Drawing for the job (mm, zero at the part's lowest x, y, z). Give positions to 0.01 mm unless a question says otherwise; leave off trailing zeros.
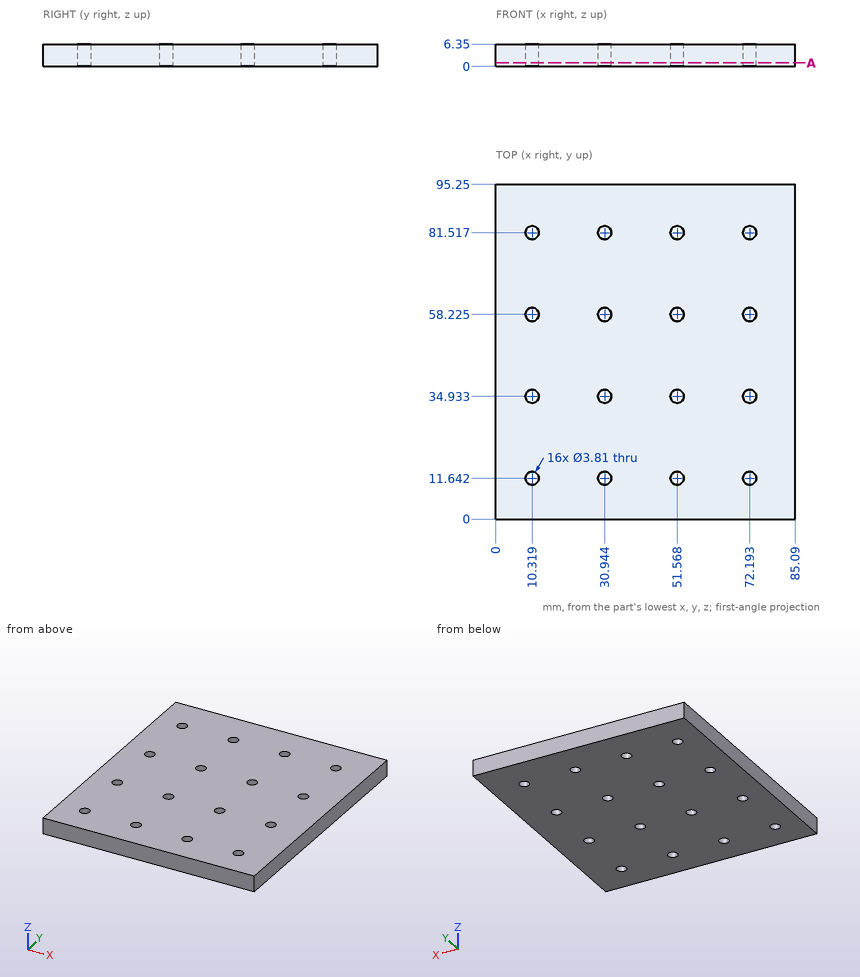
1. Slice it at A-A, the plane z = 1. State how many separate pieces and enclosed holes the cut face has, and give its area (3 significant figures).
Calculated:
separate pieces: 1
enclosed holes: 16
area: 7,920 mm2
2. Probe probe 1 along X at (y, z) = (12, 2.5) (1 decimal). List the from-to ranges inside material, lowest first.
Calculated:
probe 1: x = 0 to 8.4, 12.2 to 29.1, 32.8 to 49.7, 53.4 to 70.3, 74.1 to 85.1
3. Pin check, flat tip, straight feed: P1, Ø3, axis at x = 10.32, y = 34.93, coming from the -Z side. Stop position of the tip, or through.
Calculated:
P1: passes through
